Build history of the part. All positions in model axes, mm. Face numbers are marked on the shaded views. A direction names the side the tool comes from. Round coordinates to 2 decimals unless told otherwise and drop trailing zeros. Write each loop counter-clockwise with the first axis right and the second up, starting at its lowest first coordinate (ties: lowest second). Pieces come first, ordered by that corner, then holes. Notation, with made-up numbers: (-17.5, 66) -> (12.5, 66) arc R32 ccw to (12.5, 102) -> close; hole circle Ø11 at (80.5, 66.5). An arc over 180 degrees is marked (long way). Answer as CSV lines item,"result".
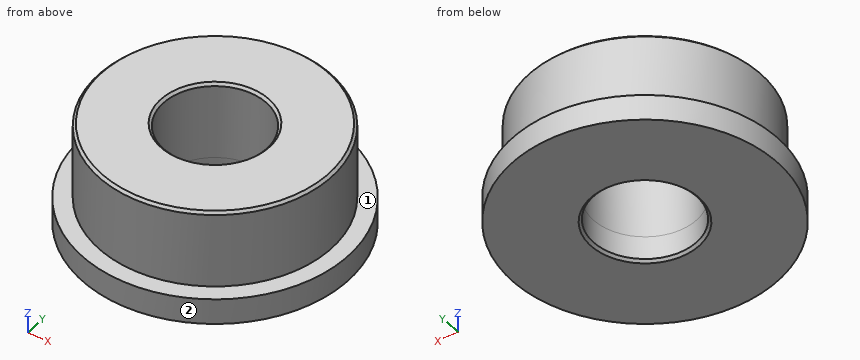
Autodesk Inventor part; units mm, degrees
ref_plane "YZ Plane" through (0, 0, 0) normal (1, 0, 0) x (0, 1, 0)
ref_plane "XZ Plane" through (0, 0, 0) normal (0, 1, 0) x (-1, 0, 0)
ref_plane "XY Plane" through (0, 0, 0) normal (0, 0, 1) x (1, 0, 0)
sketch "スケッチ1" plane through (0, 0, 0) normal (0, 0, 1) x (1, 0, 0)
  circle A0 centre (0, 0) radius 2
  circle A1 centre (0, 0) radius 4.5
  dimension "d0" = 4
  dimension "d1" = 9
extrude "押し出し1" add sketch "スケッチ1" along normal blind 3
sketch "スケッチ2" plane through (0, 0, 0) normal (0, 0, -1) x (-1, 0, 0)
  circle A0 centre (0, 0) radius 2
  circle A1 centre (0, 0) radius 5.15
  dimension "d4" = 4
  dimension "d5" = 10.3
extrude "押し出し2" add sketch "スケッチ2" along normal blind 1
chamfer "面取り1" distance 0.1 angle 45 3 edges at (-4.5, 0, 3) (-2, 0, 3) (2, 0, -1)
properties part number "ベアリング　4.9" material "ステンレス鋼"
1. Cut at A-A, the plane x = 0. Write the cut outline in (y, z).
Results found:
outline,"(-5.15, -1) -> (-2.1, -1) -> (-2, -0.9) -> (-2, 2.9) -> (-2.1, 3) -> (-4.4, 3) -> (-4.5, 2.9) -> (-4.5, 0) -> (-5.15, 0) -> close; (2, -0.9) -> (2.1, -1) -> (5.15, -1) -> (5.15, 0) -> (4.5, 0) -> (4.5, 2.9) -> (4.4, 3) -> (2.1, 3) -> (2, 2.9) -> close"
2. Which spindle directions (+Z, -Z, +X, -X, +Y, -Y) get a long thin tool onto all of the face, cutting with end or side? Do the marked faces 1 and 2. Say none if no direction does.
Results found:
face 1,"+Z"
face 2,"+Z, -Z"
3. Probe line 1 along Y through (x, z) = (0, 2.1); line 2 along Y through (x, z) = (0, -0.4); line 3 along Z through (x, y) = (4.75, -1). List the from-to ranges inside material, lowest first.
Results found:
line 1,"y = -4.5 to -2, 2 to 4.5"
line 2,"y = -5.15 to -2, 2 to 5.15"
line 3,"z = -1 to 0"
4. Cut at C-C, the plane z = 2.1. Write the cut outline in (x, y), then the cut area to 3 significant figures.
Results found:
outline,"circle Ø9 at (0, 0); hole circle Ø4 at (0, 0)"
area,"51.1 mm2"
5. Drop flat-ended pins along their axis: pin 1 Ø3.5 at (x, y) = (0, 0) entering from +Z; pin 2 Ø2 at (x, z) = (3.5, -0.5) entering from -Y; pin 3 Ø2 at (x, z) = (-3.5, 2) entering from -Y. Give the stop position or say it passes through.
Results found:
pin 1,"passes through"
pin 2,"stops at y = -4.5"
pin 3,"stops at y = -3.74"
